Input: part model. Units: mm. Frame: model coordinates. Face numbers are marked on the shaded views. A direction names the side the tool comes from. Give positions to 0.01 mm unless a question says otherwise; leave off trailing zeros. Loops run counter-clockwise (first coordinate to the right, second up) from the corner with the lowest first, then second, coordinate; pieces in that order, holes last. Notation, with made-up numbers: (-9.5, 59) -> (13.5, 59) arc R21 ccw to (13.5, 84) -> close; hole circle Ø9 at (88.25, 19). An arc over 180 degrees is marked (long way). Use CSV: the item, a comma, the result in double quotes.
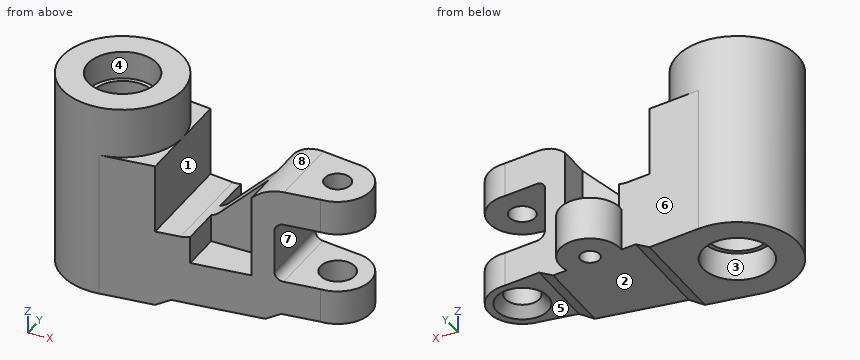
```python
from build123d import *

# Parameters (mm, degrees)
SKETCH1_R                = 7
SKETCH1_R_2              = 3.5
CYLINDER_DEPTH           = 22.85
SKETCH2_R                = 4
BORE_1_DEPTH             = 3.25
BORE_START               = -3.25
SKETCH3_R                = 4
BORE_2_DEPTH             = 3.25
ARM_DEPTH                = 17
SKETCH5_R                = 3.5
OUTER_HOLE_SURFACE_DEPTH = 6
SKETCH6_R                = 1.125
OUTER_HOLE_DEPTH         = 6
SIDE_FEATURES_DEPTH      = 22
RIB_START                = -11
SKETCH10_W               = 6.681980515
SKETCH10_H               = 4.679772507
RIB_DEPTH                = 9.5
SKETCH13_R               = 1.5
BOTTOM_HOLE_DEPTH        = 4


# Read off the part's stored shape, not the designer's step: Top Counter-sunk
with BuildPart() as part:
    # Sketch1 → Cylinder (new body)
    with BuildSketch(Plane.XY):
        with Locations(Location((0, 0, 0), (0, 0, 180))):
            Circle(SKETCH1_R)
        with Locations(Location((0, 0, 0), (0, 0, 180))):
            Circle(SKETCH1_R_2, mode=Mode.SUBTRACT)
    extrude(amount=CYLINDER_DEPTH)

    # Sketch2 → Bore 1 (cut)
    with BuildSketch(Plane.XY.offset(22.85)):
        Circle(SKETCH2_R)
    extrude(amount=-BORE_1_DEPTH, mode=Mode.SUBTRACT)

    # Sketch3 → Bore 2 (cut)
    with BuildSketch(Plane(origin=(0, 0, 0), x_dir=(-1, 0, 0), z_dir=(0, 0, -1)).offset(BORE_START)):
        with Locations(Location((0, 0, 0), (0, 0, 180))):
            Circle(SKETCH3_R)
    extrude(amount=BORE_2_DEPTH, mode=Mode.SUBTRACT)

    # Sketch4 → Arm (add)
    with BuildSketch(Plane.XY):
        with BuildLine():
            Line((0.8836803, 6.943998065), (25, 3.875))
            ThreePointArc((25, 3.875), (28.875, 0), (25, -3.875))
            Line((25, -3.875), (0.8836803, -6.943998065))
            ThreePointArc((0.8836803, -6.943998065), (7, 0), (0.8836803, 6.943998065))
        make_face()
    extrude(amount=ARM_DEPTH)

    # Sketch5 → Outer Hole surface (add)
    with BuildSketch(Plane(origin=(0, 0, 0), x_dir=(-1, 0, 0), z_dir=(0, 0, -1))):
        with Locations((-14, 6)):
            Circle(SKETCH5_R)
    extrude(amount=-OUTER_HOLE_SURFACE_DEPTH)

    # Sketch6 → Outer hole (cut)
    with BuildSketch(Plane(origin=(0, 0, 0), x_dir=(-1, 0, 0), z_dir=(0, 0, -1))):
        with Locations((-14, 6)):
            Circle(SKETCH6_R)
    extrude(amount=-OUTER_HOLE_DEPTH, mode=Mode.SUBTRACT)

    # Sketch8 → side Features (cut)
    with BuildSketch(Plane(origin=(0, 10, 0), x_dir=(1, 0, 0), z_dir=(0, 1, 0))):
        with BuildLine():
            Line((21, -6), (40, -6))
            Line((40, -6), (40, -13))
            Line((40, -13), (21, -13))
            ThreePointArc((21, -13), (20.292893219, -12.707106781), (20, -12))
            Line((20, -12), (20, -7))
            ThreePointArc((20, -7), (20.292893219, -6.292893219), (21, -6))
        make_face()
        with BuildLine():
            Line((7, -19), (7, -9))
            Line((7, -9), (9.757359313, -9))
            ThreePointArc((9.757359313, -9), (10.90540961, -9.228361402), (11.878679656, -9.878679656))
            Line((11.878679656, -9.878679656), (17.535533906, -15.535533906))
            ThreePointArc((17.535533906, -15.535533906), (19.15765065, -16.619397663), (21.071067812, -17))
            Line((21.071067812, -17), (27, -17))
            Line((27, -17), (27, -19))
            Line((27, -19), (7, -19))
        make_face()
        Polygon((7, 0), (8.732050808, -1), (19, -1), (20.732050808, -2), (40, -2), (40, 0), align=None)
    extrude(amount=-SIDE_FEATURES_DEPTH, mode=Mode.SUBTRACT)

    # Sketch10 → Rib (cut)
    with BuildSketch(Plane.XY.offset(17).offset(RIB_START)):
        with Locations((14.159009743, 3.339886254)):
            Rectangle(SKETCH10_W, SKETCH10_H)
        with Locations((14.159009743, -3.339886254)):
            Rectangle(SKETCH10_W, SKETCH10_H)
    extrude(amount=RIB_DEPTH, mode=Mode.SUBTRACT)

    # Top Counter-sunk outline → Top Counter-sunk (revolve, cut)
    with BuildSketch(Plane(origin=(25, 0, 0), x_dir=(1, 0, 0), z_dir=(0, -1, 0))):
        Polygon((2, 3.150368407), (2, 6), (0, 6), (0, 2), (3, 2), align=None)
    revolve(axis=Axis((25, 0, 0), (0, 0, 1)), mode=Mode.SUBTRACT)

    # Sketch13 → Bottom hole (cut)
    with BuildSketch(Plane.XY.offset(17)):
        with Locations((25, 0)):
            Circle(SKETCH13_R)
    extrude(amount=-BOTTOM_HOLE_DEPTH, mode=Mode.SUBTRACT)


solid = part.part
```
1) Section query D-D (y = 0.5). Give the number of separate pieces and of enclosed holes in the cut face, then the cut area to 3 significant figures.
From the geometry:
separate pieces,"4"
enclosed holes,"0"
area,"342 mm^2"
2) Contact query for flat-ended pins moving along their axis: pin 1 (4 mm diameter, centred on x = 8, y = -3, fed in from -Z); pin 2 (6.5 mm diameter, centred on x = 25, y = 0, fed in from -Z); pin 3 (5 mm diameter, centred on x = 13, y = -4, fed in from +Z); pin 4 (2 mm diameter, centred on x = 15.5, z = 10.5, fed in from +Y). Output: stop coordinate, or through.
From the geometry:
pin 1,"stops at z = 0"
pin 2,"stops at z = 2"
pin 3,"stops at z = 9.19"
pin 4,"stops at y = 1"
3) Section query C-C (x = 5). Return loops of the section in (y, z).
From the geometry:
outline,"(-6.42, 0) -> (6.42, 0) -> (6.42, 17) -> (4.9, 17) -> (4.9, 22.85) -> (-4.9, 22.85) -> (-4.9, 17) -> (-6.42, 17) -> close"
4) Section query A-A (x = 14). Return loops of the section in (y, z) (3 decimals), then the cut area to 3 significant figures.
From the geometry:
outline,"(-5.275, 1) -> (4.875, 1) -> (4.875, 6) -> (1, 6) -> (1, 12) -> (-1, 12) -> (-1, 6) -> (-5.275, 6) -> close; (7.125, 1) -> (9.5, 1) -> (9.5, 6) -> (7.125, 6) -> close"
area,"74.6 mm^2"
5) Reachability of the marked faces 1, 2, 3 and 4 from +Z, -Z, +X, -X, +Y, -Y: full face, straight path, thin tool, end or side. Return the list, or none.
From the geometry:
face 1,"+Z, +Y, -Y"
face 2,"-Z, +X, +Y, -Y"
face 3,"-Z"
face 4,"+Z"
6) Mould query, pull axis Z, two halves, no side actions, for the marked faces 5, 6, 7 and 8. Classes: pulls with the +Z half, pulls with the -Z half, needs draft (parallel to the pull), parting line crosses it, or undercut.
From the geometry:
face 5,"pulls with the -Z half"
face 6,"needs draft"
face 7,"undercut"
face 8,"pulls with the +Z half"
7) Section query B-B (z = 3.75). Return loops of the section in (x, y) (3 decimals), then the cut area to 3 significant figures.
From the geometry:
outline,"(0.884, -6.944) -> (25, -3.875) arc R3.875 ccw to (25, 3.875) -> (17.307, 4.854) arc R3.5 ccw (long way) to (10.511, 5.719) -> (0.884, 6.944) arc R7 ccw (long way) to start; hole circle Ø7 at (0, 0); hole circle Ø2.25 at (14, 6); hole circle Ø4 at (25, 0)"
area,"343 mm^2"
8) Ray query, line 1 (Y direction, x = 0, z = 21.05); line 2 (Y direction, x = 25, z = 15.75) (3 decimals); line 3 (X direction, y = 2, z = 7.5). Return the intervals inside material, ascending.
From the geometry:
line 1,"y = -7 to -4, 4 to 7"
line 2,"y = -3.875 to -1.5, 1.5 to 3.875"
line 3,"x = -6.71 to -2.87, 2.87 to 10.82, 17.5 to 20"
